```python
from build123d import *

# Parameters (mm, degrees)
BOSS_EXTRUDE1_DEPTH = 5
SKETCH3_R           = 0.75
CUT_EXTRUDE1_DEPTH  = 4
SKETCH4_R           = 1
CUT_EXTRUDE2_DEPTH  = 4
CHAMFER1_SIZE       = 1


with BuildPart() as part:
    # Sketch2 → Boss-Extrude1 (new body)
    with BuildSketch(Plane(origin=(0, 0, 0), x_dir=(1, 0, 0), z_dir=(0, 1, 0))):
        Polygon((0, 0), (0, 15.470692064), (-9.5, 45), (-9.5, 68), (-12.5, 68), (-12.5, 44.529307936), (-3, 15), (-3, 0), align=None)
    extrude(amount=BOSS_EXTRUDE1_DEPTH)

    # Sketch3 → Cut-Extrude1 (cut, through all)
    with BuildSketch(Plane.ZY.offset(3)):
        with Locations((-2.5, 2.5)):
            Circle(SKETCH3_R)
    extrude(amount=-CUT_EXTRUDE1_DEPTH, mode=Mode.SUBTRACT)

    # Sketch4 → Cut-Extrude2 (cut, through all)
    with BuildSketch(Plane(origin=(-9.5, 0, 0), x_dir=(0, 0, -1), z_dir=(1, 0, 0))):
        with Locations((65.5, 2.5)):
            Circle(SKETCH4_R)
    extrude(amount=-CUT_EXTRUDE2_DEPTH, mode=Mode.SUBTRACT)

    # Chamfer1
    chamfer1_edges = [part.edges().sort_by_distance(p)[0] for p in [
        (-1.5, 0, 0),
        (-11, 5, -68),
        (-1.5, 5, 0),
        (-11, 0, -68),
    ]]
    chamfer(chamfer1_edges, length=CHAMFER1_SIZE)


solid = part.part
```
Check sheet for the modelled part. Datum: model origin and axes. Units: mm. A direction names the side the tool comes from. Coordinates: 2 decimals unless noted, no trailing zeros. Order: outer loops, then holes, each group sorted by start corner. A loop starts at its lowest first (then second) coordinate and runs counter-clockwise, first axis right, second up. Notation, with made-up numbers: M -26,11 L 30,11 A23 ccw 30,29 Z; hole C 55.25,29.25 d1. An arc over 180 degrees is marked long. Write each question's results on one line, items separated by ' | '. Start each with the question number.
1. Cross-section at C-C on z = -2.5. Record the cut outline in (x, y).
2. Material ranges on probe 1 along Y at (x, z) = (-11.1, -65.5); probe 2 along Y at (x, z) = (-1.6, -2.5); probe 3 along X at (y, z) = (3.95, -12.5), recorded low to high.
3. Cross-section at D-D on z = -30. Record the cut outline in (x, y).
4. Cross-section at B-B on y = 2.5. Record the cut outline in (x, z), and give its area (3 significant figures).
5. Mould release check, pull along Y, two halves, no side actions. Record for faces 4 (the face through (-7, 0, -34)), 5 (the face through (-11, 2, -68)), 6 (the face through (-1.521, 2.044, -3.095)): +Y half, -Y half, draft (parallel to the pull), parting line (faces both ways), or undercut.
6. Access from +Z, -Z, +X, -X, +Y, -Y to the whole of each face (thin tool, end or side, straight path). Record for faces 1 (the face through (-9.5, 2, -56)), 2 (the face through (-3, 2, -8)), 3 (the face through (-7, 5, -34)).
7. Go/stop test with flat-tipped pins: P1, Ø2, axis at x = -9, y = 0.5, coming from the -Z side; P2, Ø1, axis at y = 1, z = -31, coming from the +X side; P3, Ø3, axis at y = 3, z = -23.5, coming from the -X side. Record where each tip stops, or that it passes through.
8. Cross-section at A-A on z = -65.5. Record the cut outline in (x, y).
Checks:
1) outline: M -3,0 L 0,0 L 0,1.75 L -3,1.75 Z; M -3,3.25 L 0,3.25 L 0,5 L -3,5 Z
2) probe 1: y = 0 to 1.5, 3.5 to 5 | probe 2: y = 0 to 1.75, 3.25 to 5 | probe 3: x = -3 to 0
3) outline: M -7.83,0 L -4.67,0 L -4.67,5 L -7.83,5 Z
4) outline: M -12.5,-68 L -9.5,-68 L -9.5,-66.5 L -12.5,-66.5 Z; M -12.5,-64.5 L -9.5,-64.5 L -9.5,-45 L 0,-15.47 L 0,-3.25 L -3,-3.25 L -3,-15 L -12.5,-44.53 Z; M -3,-1.75 L 0,-1.75 L 0,0 L -3,0 Z | area: 198 mm²
5) face 4: -Y half | face 5: draft | face 6: undercut
6) face 1: -Z, +X, +Y, -Y | face 2: +Z, -X, +Y, -Y | face 3: +Z, -Z, +X, -X, +Y
7) P1: stops at z = -68 | P2: stops at x = -4.84 | P3: stops at x = -6.22
8) outline: M -12.5,0 L -9.5,0 L -9.5,1.5 L -12.5,1.5 Z; M -12.5,3.5 L -9.5,3.5 L -9.5,5 L -12.5,5 Z
